For this review, use the dimensioned drawing (mm, ordinates from the lowest corner) and the shaded views. Coordinates: 2 decimals unless noted, no trailing zeros. Loops run counter-clockwise (first coordinate to the right, second up) from the corner with the lowest first, then second, coordinate; pieces in that order, holes last. Notation, with made-up numbers: (64.5, 25.25) - (103.5, 25.25) arc R12 ccw to (103.5, 35.25) - close; hole circle Ø8 at (-12.75, 11). An arc over 180 degrees is marked (long way). Answer in a Markdown table with one row per item. Add a question column.
(1) For line 1 along X through (y, z) = (41, 279.5); line 2 along Y through (x, z) = (34, 491.5); line 3 along Y through (x, z) = (616.5, 119.5), list the stretches that pass through material, from the lowest coordinate up.
(2) We need section C-C on x = 432. Write out the cut boundary in (y, z).
(3) We need section B-B on z = 333. Write out the cut boundary in (x, y).
(4) Mouldability with a two-part tool opening along X and no side actions: class the marked faces 1 and 2 as +X half, -X half, draft (parallel to the pull), parting line (faces both ways), or undercut.
(5) We need section A-A on y = 22.5. Write out the cut boundary in (x, z), plus the area to 3 significant figures.
(6) For P1, Ø8, axis at y = 53.5, z = 481.5, coming from the -X side; P2, Ø15, axis at x = 16, z = 335, coming from the -Y side, all flat-tipped, find the tip position at first contact; note any pin that passes through.
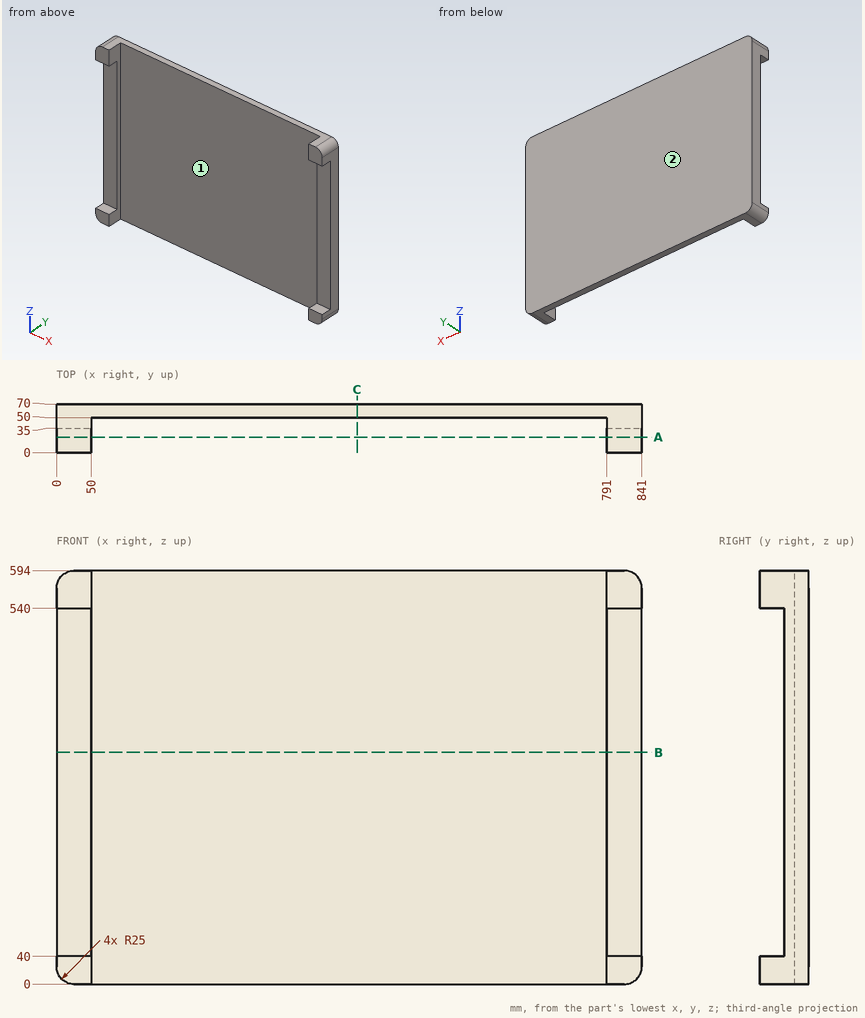
Outcome:
| question | item | result |
|---|---|---|
| 1 | line 1 | 0 to 50, 791 to 841 |
| 1 | line 2 | 35 to 70 |
| 1 | line 3 | 50 to 70 |
| 2 | outline | (50, 0) - (70, 0) - (70, 594) - (50, 594) - close |
| 3 | outline | (0, 35) - (50, 35) - (50, 50) - (791, 50) - (791, 35) - (841, 35) - (841, 70) - (0, 70) - close |
| 4 | face 1 | undercut |
| 4 | face 2 | draft |
| 5 | outline | (0, 25) arc R25 ccw to (25, 0) - (50, 0) - (50, 40) - (0, 40) - close; (0, 540) - (50, 540) - (50, 594) - (25, 594) arc R25 ccw to (0, 569) - close; (791, 0) - (816, 0) arc R25 ccw to (841, 25) - (841, 40) - (791, 40) - close; (791, 540) - (841, 540) - (841, 569) arc R25 ccw to (816, 594) - (791, 594) - close |
| 5 | area | 8,860 mm² |
| 6 | P1 | x = 0 |
| 6 | P2 | y = 35 |
